```python
from build123d import *

# Parameters (mm, degrees)
SKETCH_1_W           = 96.5
SKETCH_1_H           = 35
EXTRUDE_1_DEPTH      = 6
SKETCH_2_W           = 82
SKETCH_2_H           = 24
CUT_EXTRUDE_1_DEPTH  = 5
CUT_EXTRUDE_2_DEPTH  = 6
CUT_EXTRUDE_3_DEPTH  = 2.1
FILLET_1_R           = 1
CHAMFER_1_SIZE       = 0.6
CHAMFER_2_SIZE       = 0.4
FILLET_2_R           = 0.2
SKETCH_5_W           = 10.55
SKETCH_5_H           = 11
CUT_EXTRUDE_5_DEPTH  = 103.725167316
CHAMFER_3_SIZE       = 0.6
CHAMFER_4_SIZE       = 0.6
SKETCH_6_W           = 1
SKETCH_6_H           = 9.5
CUT_EXTRUDE_6_DEPTH  = 3
CHAMFER_5_SIZE       = 1
CHAMFER_6_SIZE       = 1
SKETCH_7_W           = 6.2
SKETCH_7_H           = 2.1
CUT_EXTRUDE_7_DEPTH  = 6
SKETCH_8_R           = 1.2
CUT_EXTRUDE_8_DEPTH  = 103.736994311
SKETCH_11_R          = 1.2
CUT_EXTRUDE_9_DEPTH  = 103.826309863
SKETCH_11_3_R        = 2.05
CUT_EXTRUDE_10_DEPTH = 2


with BuildPart() as part:
    # 草图1 → 凸台-拉伸1 (new body)
    with BuildSketch(Plane(origin=(0, 0, 0), x_dir=(1, 0, 0), z_dir=(0, 1, 0))):
        with Locations((48.25, 17.5)):
            Rectangle(SKETCH_1_W, SKETCH_1_H)
    extrude(amount=EXTRUDE_1_DEPTH)

    # 草图2 → 切除-拉伸1 (cut)
    with BuildSketch(Plane(origin=(0, 6, 0), x_dir=(1, 0, 0), z_dir=(0, 1, 0))):
        with Locations((43, 19)):
            Rectangle(SKETCH_2_W, SKETCH_2_H)
    extrude(amount=-CUT_EXTRUDE_1_DEPTH, mode=Mode.SUBTRACT)

    # 草图3 → 切除-拉伸2 (cut)
    with BuildSketch(Plane.XY):
        Polygon((96.5, 6), (96.5, 0), (0, 0), (0, 6), (2.1, 6), (2.1, 2.1), (94.4, 2.1), (94.4, 6), align=None)
    extrude(amount=-CUT_EXTRUDE_2_DEPTH, mode=Mode.SUBTRACT)

    # 草图4 → 切除-拉伸3 (cut)
    with BuildSketch(Plane.XZ):
        Polygon((0, -32.2), (85.95, -32.2), (85.95, -24), (86, -24), (96.5, -24), (96.5, -35), (0, -35), align=None)
    extrude(amount=-CUT_EXTRUDE_3_DEPTH, mode=Mode.SUBTRACT)

    # 圆角1
    fillet_1_edges = [part.edges().sort_by_distance(p)[0] for p in [
        (85.95, 1.05, -32.2),
    ]]
    fillet(fillet_1_edges, radius=FILLET_1_R)

    # 倒角1
    chamfer_1_edges = [part.edges().sort_by_distance(p)[0] for p in [
        (91.225, 0, -24),
        (85.95, 0, -27.6),
        (42.475, 0, -32.2),
        (85.657106781, 0, -31.907106781),
    ]]
    chamfer(chamfer_1_edges, length=CHAMFER_1_SIZE)

    # 倒角2
    chamfer_2_edges = [part.edges().sort_by_distance(p)[0] for p in [
        (96.5, 0, -14.7),
        (0, 0, -18.8),
    ]]
    chamfer(chamfer_2_edges, length=CHAMFER_2_SIZE)

    # 圆角2
    fillet_2_edges = [part.edges().sort_by_distance(p)[0] for p in [
        (96.1, 0, -14.7),
        (0.4, 0, -18.8),
        (96.5, 0.4, -14.9),
        (0, 0.4, -19),
    ]]
    fillet(fillet_2_edges, radius=FILLET_2_R)

    # 草图5 → 切除-拉伸5 (cut, through all)
    with BuildSketch(Plane.XZ.offset(-2.1)):
        with Locations((91.225, -29.5)):
            Rectangle(SKETCH_5_W, SKETCH_5_H)
    extrude(amount=-CUT_EXTRUDE_5_DEPTH, mode=Mode.SUBTRACT)

    # 倒角3
    chamfer_3_edges = [part.edges().sort_by_distance(p)[0] for p in [
        (91.225, 6, -24),
        (2.1, 2.1, -3),
        (94.4, 2.1, -3),
    ]]
    chamfer(chamfer_3_edges, length=CHAMFER_3_SIZE)

    # 倒角4
    chamfer_4_edges = [part.edges().sort_by_distance(p)[0] for p in [
        (42.975, 2.1, -35),
    ]]
    chamfer(chamfer_4_edges, length=CHAMFER_4_SIZE)

    # 草图6 → 切除-拉伸6 (cut)
    with BuildSketch(Plane(origin=(0, 6, 0), x_dir=(1, 0, 0), z_dir=(0, 1, 0))):
        with Locations((1.5, 26.25)):
            Rectangle(SKETCH_6_W, SKETCH_6_H)
    extrude(amount=-CUT_EXTRUDE_6_DEPTH, mode=Mode.SUBTRACT)

    # 倒角5
    chamfer_5_edges = [part.edges().sort_by_distance(p)[0] for p in [
        (2, 3, -26.25),
    ]]
    chamfer(chamfer_5_edges, length=CHAMFER_5_SIZE - 0.0001)  # a hair under: the kernel refuses the full size

    # 倒角6
    chamfer_6_edges = [part.edges().sort_by_distance(p)[0] for p in [
        (2, 4.00005, -21.5),
    ]]
    chamfer(chamfer_6_edges, length=CHAMFER_6_SIZE - 0.0001)  # a hair under: the kernel refuses the full size

    # 草图7 → 切除-拉伸7 (cut)
    with BuildSketch(Plane.XY):
        with Locations((66.5, 3.15)):
            Rectangle(SKETCH_7_W, SKETCH_7_H)
        with Locations((30, 3.15)):
            Rectangle(SKETCH_7_W, SKETCH_7_H)
    extrude(amount=-CUT_EXTRUDE_7_DEPTH, mode=Mode.SUBTRACT)

    # 草图8 → 切除-拉伸8 (cut, through all)
    with BuildSketch(Plane.XZ.offset(-4.2)):
        with Locations(Location((66.5, -3, 0), (0, 0, 270))):
            Circle(SKETCH_8_R)
        with Locations(Location((30, -3, 0), (0, 0, 270))):
            Circle(SKETCH_8_R)
    extrude(amount=-CUT_EXTRUDE_8_DEPTH, mode=Mode.SUBTRACT)

    # 草图11 → 切除-拉伸9 (cut, through all)
    with BuildSketch(Plane.XZ):
        with Locations(Location((93.5, -19, 0), (0, 0, 270))):
            Circle(SKETCH_11_R)
    extrude(amount=-CUT_EXTRUDE_9_DEPTH, mode=Mode.SUBTRACT)

    # 草图11<3> → 切除-拉伸10 (cut)
    with BuildSketch(Plane.XZ):
        with Locations(Location((93.5, -19, 0), (0, 0, 270))):
            Circle(SKETCH_11_3_R)
    extrude(amount=-CUT_EXTRUDE_10_DEPTH, mode=Mode.SUBTRACT)


solid = part.part
```
Geometry: final body of the model. Coordinates: model frame, mm. A direction names the side the tool comes from. Coordinates: 2 decimals unless noted, no trailing zeros. Order: outer loops, then holes, each group sorted by start corner. A loop starts at its lowest first (then second) coordinate and runs counter-clockwise, first axis right, second up. Notation, with made-up numbers: (-9.5, 80.25) - (3.5, 80.25) arc R26 ccw to (3.5, 105.25) - close; hole circle Ø2 at (81, -16.75). An arc over 180 degrees is marked (long way). Return JSON: item names as keys, results as strings. Group by question number.
1. Pin query (flat end, axial travel): pin 1 (2.5 mm diameter, centred on x = 30, z = -33, fed in from -Y); pin 2 (3.5 mm diameter, centred on y = 4.5, z = -28, fed in from +X); pin 3 (3.5 mm diameter, centred on x = 93.5, z = -19, fed in from -Y); pin 4 (1.9 mm diameter, centred on x = 93.5, z = -19, fed in from +Y). Return the tip coordinate at first contact, or that it passes through.
2. Pull-direction query (X, two-part tool) for faces 5 (the face through (48, 0, -19)), 6 (the face through (85.95, 3, -29)), 7 (the face through (92, 2, -19)); classes: pulls with the +X half, pulls with the -X half, needs draft (parallel to the pull), parting line crosses it, or undercut.
3. Cut plane C-C (x = 30). Output: boundary loops of the cut face in (y, z).
4. Cut plane A-A (z = -3). Output: boundary loops of the cut face in (x, y).
5. Cut plane B-B (z = -19). Output: boundary loops of the cut face in (x, y), plus the area to 3 significant figures.
6. Cut plane D-D (x = 10). Output: boundary loops of the cut face in (y, z).
7. Material intervals for line 1 along X through (y, z) = (5.25, -3); line 2 along X through (y, z) = (2.25, -9.5); line 3 along Z through (x, y) = (66.5, 5.65), sorted ascending. Write a range as [from, to].
8. Set-up query: faces 1 (the face through (26.9, 3, -3)), 2 (the face through (91, 3, -24)), 3 (the face through (2, 3, -16)), 4 (the face through (15, 2.1, -3)). Return all of +Z, -Z, +X, -X, +Y, -Y with unobstructed straight access to the full face (end or side cutting, diameter ignored); none if empty.
Resolved:
{
 "1": {"pin 1": "stops at y = 0.15", "pin 2": "stops at x = 85.95", "pin 3": "stops at y = 2", "pin 4": "passes through"},
 "2": {"face 5": "needs draft", "face 6": "pulls with the +X half", "face 7": "undercut"},
 "3": {"outline": "(0, -31.6) - (0.6, -32.2) - (2.1, -32.2) - (2.1, -34.4) - (2.7, -35) - (6, -35) - (6, -31) - (1, -31) - (1, -7) - (6, -7) - (6, -4.2) - (4.2, -4.2) - (4.2, -6) - (0, -6) - close; (4.2, -1.8) - (6, -1.8) - (6, 0) - (4.2, 0) - close"},
 "4": {"outline": "(2.1, 2.7) - (2.7, 2.1) - (26.9, 2.1) - (26.9, 4.2) - (28.8, 4.2) - (28.8, 6) - (2.1, 6) - close; (31.2, 4.2) - (33.1, 4.2) - (33.1, 2.1) - (63.4, 2.1) - (63.4, 4.2) - (65.3, 4.2) - (65.3, 6) - (31.2, 6) - close; (67.7, 4.2) - (69.6, 4.2) - (69.6, 2.1) - (93.8, 2.1) - (94.4, 2.7) - (94.4, 6) - (67.7, 6) - close"},
 "5": {"outline": "(0, 0.48) arc R0.2 ccw to (0.06, 0.34) - (0.34, 0.06) arc R0.2 ccw to (0.48, 0) - (91.45, 0) - (91.45, 2) - (92.3, 2) - (92.3, 6) - (84, 6) - (84, 1) - (2, 1) - (2, 6) - (0, 6) - close; (94.7, 2) - (95.55, 2) - (95.55, 0) - (96.02, 0) arc R0.2 ccw to (96.16, 0.06) - (96.44, 0.34) arc R0.2 ccw to (96.5, 0.48) - (96.5, 6) - (94.7, 6) - close", "area": "151 mm²"},
 "6": {"outline": "(0, -31.6) - (0.6, -32.2) - (2.1, -32.2) - (2.1, -34.4) - (2.7, -35) - (6, -35) - (6, -31) - (1, -31) - (1, -7) - (6, -7) - (6, 0) - (2.1, 0) - (2.1, -6) - (0, -6) - close"},
 "7": {"line 1": "x = [2.1, 28.8], [31.2, 65.3], [67.7, 94.4]", "line 2": "x = [0, 2], [84, 96.5]", "line 3": "z = [-35, -31], [-7, -4.2], [-1.8, 0]"},
 "8": {"face 1": "+Z, -Y", "face 2": "-Z, +X, +Y, -Y", "face 3": "+Y", "face 4": "+Z, +X, -X, -Y"}
}
